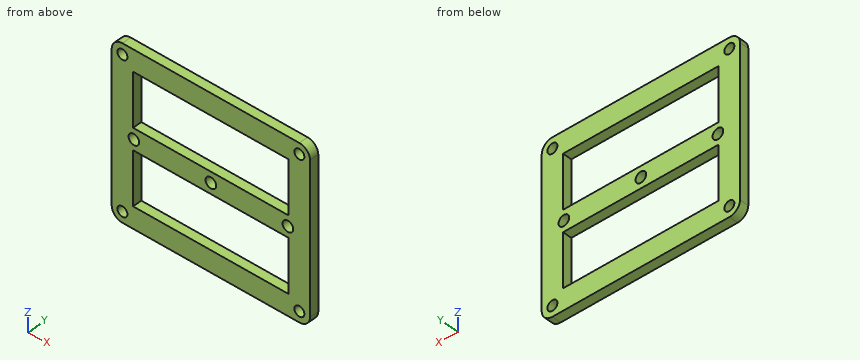
from build123d import *

# Parameters (mm, degrees)
SKETCH1_W           = 65
SKETCH1_H           = 56
SKETCH1_R           = 1.65
SKETCH1_W_2         = 51
SKETCH1_H_2         = 17.5
BOSS_EXTRUDE1_DEPTH = 3
FILLET1_R           = 3.5
CUT_EXTRUDE1_REACH  = 82.917
SKETCH2_R           = 1.75


with BuildPart() as part:
    # Sketch1 → Boss-Extrude1 (new body)
    with BuildSketch(Plane(origin=(0, 0, 0), x_dir=(1, 0, 0), z_dir=(0, 1, 0))):
        with Locations((29, 24.5)):
            Rectangle(SKETCH1_W, SKETCH1_H)
        with Locations(Location((0, 49, 0), (0, 0, 270))):
            Circle(SKETCH1_R, mode=Mode.SUBTRACT)
        with Locations(Location((58, 49, 0), (0, 0, 270))):
            Circle(SKETCH1_R, mode=Mode.SUBTRACT)
        with Locations(Location((58, 0, 0), (0, 0, 270))):
            Circle(SKETCH1_R, mode=Mode.SUBTRACT)
        with Locations(Location((0, 0, 0), (0, 0, 270))):
            Circle(SKETCH1_R, mode=Mode.SUBTRACT)
        with Locations((29, 36.75)):
            Rectangle(SKETCH1_W_2, SKETCH1_H_2, mode=Mode.SUBTRACT)
        with Locations((29, 12.25)):
            Rectangle(SKETCH1_W_2, SKETCH1_H_2, mode=Mode.SUBTRACT)
    extrude(amount=BOSS_EXTRUDE1_DEPTH)

    # Fillet1
    fillet1_edges = [part.edges().sort_by_distance(p)[0] for p in [
        (-3.5, 1.5, -52.5),
        (61.5, 1.5, -52.5),
        (61.5, 1.5, 3.5),
        (-3.5, 1.5, 3.5),
    ]]
    fillet(fillet1_edges, radius=FILLET1_R)

    # Sketch2 → Cut-Extrude1 (cut, up to next)
    with BuildSketch(Plane(origin=(0, 3, 0), x_dir=(1, 0, 0), z_dir=(0, 1, 0)), mode=Mode.PRIVATE) as cut_extrude1_sk1:
        with Locations(Location((3.75, 24.5, 0), (0, 0, 270))):
            Circle(SKETCH2_R)
    cut_extrude1_tool1 = extrude(cut_extrude1_sk1.sketch, amount=-CUT_EXTRUDE1_REACH, mode=Mode.PRIVATE) & part.part
    # Sketch2 → Cut-Extrude1 (cut, up to next)
    with BuildSketch(Plane(origin=(0, 3, 0), x_dir=(1, 0, 0), z_dir=(0, 1, 0)), mode=Mode.PRIVATE) as cut_extrude1_sk2:
        with Locations(Location((29, 24.5, 0), (0, 0, 270))):
            Circle(SKETCH2_R)
    cut_extrude1_tool2 = extrude(cut_extrude1_sk2.sketch, amount=-CUT_EXTRUDE1_REACH, mode=Mode.PRIVATE) & part.part
    # Sketch2 → Cut-Extrude1 (cut, up to next)
    with BuildSketch(Plane(origin=(0, 3, 0), x_dir=(1, 0, 0), z_dir=(0, 1, 0)), mode=Mode.PRIVATE) as cut_extrude1_sk3:
        with Locations(Location((54.25, 24.5, 0), (0, 0, 270))):
            Circle(SKETCH2_R)
    cut_extrude1_tool3 = extrude(cut_extrude1_sk3.sketch, amount=-CUT_EXTRUDE1_REACH, mode=Mode.PRIVATE) & part.part
    add(cut_extrude1_tool1.solids().sort_by_distance((3.75, 3, -24.5))[0], mode=Mode.SUBTRACT)
    add(cut_extrude1_tool2.solids().sort_by_distance((29, 3, -24.5))[0], mode=Mode.SUBTRACT)
    add(cut_extrude1_tool3.solids().sort_by_distance((54.25, 3, -24.5))[0], mode=Mode.SUBTRACT)


solid = part.part
Input: part model. Units: mm. Frame: model coordinates. Coordinates: 2 decimals unless noted, no trailing zeros. Loops run counter-clockwise (first coordinate to the right, second up) from the corner with the lowest first, then second, coordinate; pieces in that order, holes last. Notation, with made-up numbers: (21.25, 1.25) - (64.25, 1.25) arc R20 cw to (64.25, 37.25) - close; hole circle Ø2 at (-30.75, 30.25). An arc over 180 degrees is marked (long way). Answer in a Markdown table with one row per item. Add a question column.
Item 1: Section query B-B on y = 2.1. State how many separate pieces and enclosed holes the cut face has, then the cut area to 3 significant figures.
Item 2: Section query A-A on z = -36. Return the cut outline in (x, y).
Item 3: Section query C-C on x = 12. Return the cut outline in (y, z).
Item 4: Line query: line 1 along X through (y, z) = (1.8, -49); line 2 along Z through (x, y) = (27, 1.55); line 3 along X through (y, z) = (0.9, -24.5). Output: solid intervals per line, ascending. Write a range as [from, to].
Recorded:
| question | item | result |
|---|---|---|
| 1 | separate pieces | 1 |
| 1 | enclosed holes | 9 |
| 1 | area | 1,780 mm^2 |
| 2 | outline | (-3.5, 0) - (3.5, 0) - (3.5, 3) - (-3.5, 3) - close; (54.5, 0) - (61.5, 0) - (61.5, 3) - (54.5, 3) - close |
| 3 | outline | (0, -52.5) - (3, -52.5) - (3, -45.5) - (0, -45.5) - close; (0, -28) - (3, -28) - (3, -21) - (0, -21) - close; (0, -3.5) - (3, -3.5) - (3, 3.5) - (0, 3.5) - close |
| 4 | line 1 | [-3.5, -1.65], [1.65, 56.35], [59.65, 61.5] |
| 4 | line 2 | [-52.5, -45.5], [-28, -21], [-3.5, 3.5] |
| 4 | line 3 | [-3.5, 2], [5.5, 27.25], [30.75, 52.5], [56, 61.5] |
